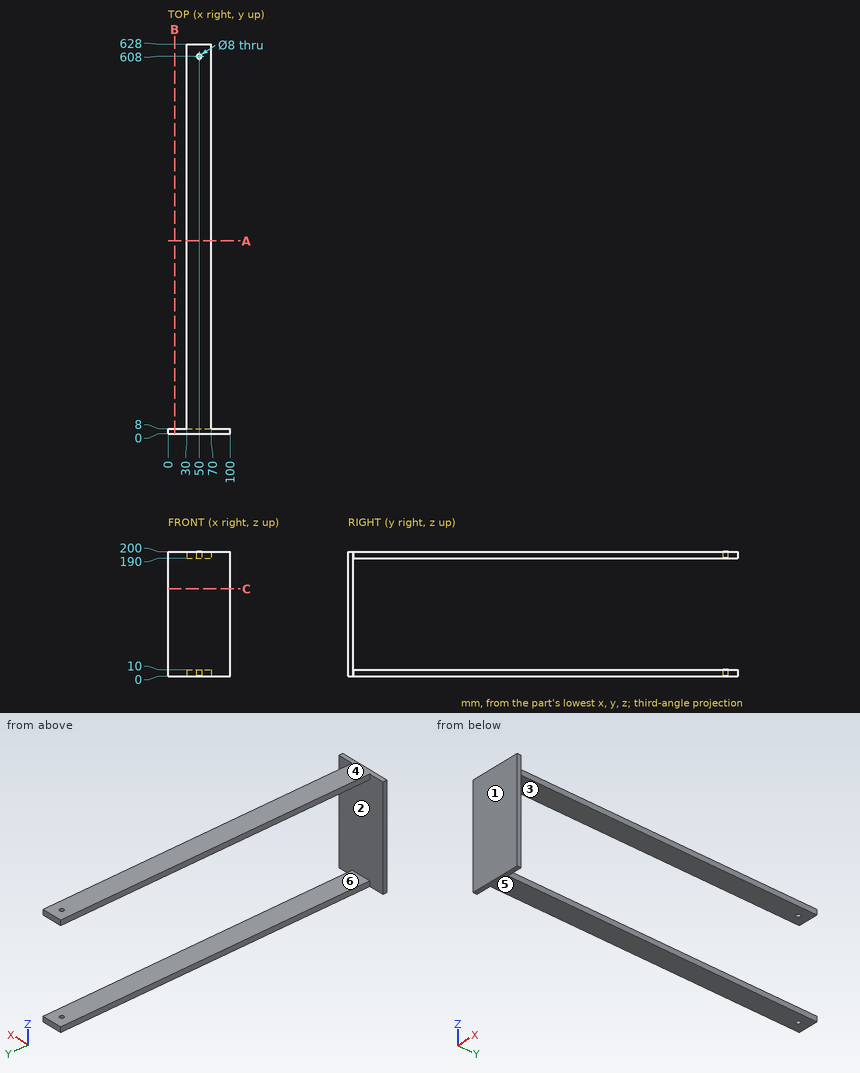
Check sheet for the drawn part. Datum: minimum x, y, z corner. Units: mm. A direction names the side the tool comes from. Round coordinates to 2 decimals unless told otherwise and drop trailing zeros. Order: outer loops, then holes, each group sorted by start corner. A loop starts at its lowest first (then second) coordinate and runs counter-clockwise, first axis right, second up. Notation, with made-up numbers: (25.25, 7.5) -> (83.25, 7.5) arc R28 ccw to (83.25, 25.5) -> close; hole circle Ø5 at (-40, 57). An arc over 180 degrees is marked (long way). Put each result on its own line as item: value. Start each with the question number.
(1) Material ranges on line 1 along Z through (x, y) = (59, 138); line 2 along Y through (x, z) = (50, 5); line 3 along Y through (x, z) = (25, 168.5), recorded low to high.
(2) Tool access check on the marked faces 5 and 6. Record the directions out of +Z, -Z, +X, -X, +Y, -Y that give a thin tool (end or side, any length) a straight path to the whole face; none if there is none.
(3) Draft check along Z on the marked faces 1, 2, 3 and 4. Enter one of: +Z half, -Z half, draft (parallel to the pull), parting line (faces both ways), or undercut.
(4) Section check A-A (y = 311). Enter the section's corners in (x, z).
(5) Depth check by flat-ended pin: pin 1 Ø1.5 at (x, z) = (54, 97.5) entering from +Y; pin 2 Ø5 at (y, z) = (400.5, 5) entering from -X; pin 3 Ø8 at (y, z) = (413, 195) entering from +X. Enter the tip coordinate at first touch or a pass-through.
(6) Section check B-B (x = 10.5). Enter the section's corners in (y, z).
(7) Section check C-C (z = 140.5). Enter the section's corners in (x, y).
Completed:
1. line 1: z = 0 to 10, 190 to 200
1. line 2: y = 0 to 604, 612 to 628
1. line 3: y = 0 to 8
2. face 5: -Z, +X, -X, +Y, -Y
2. face 6: +X, -X, +Y
3. face 1: draft
3. face 2: undercut
3. face 3: undercut
3. face 4: +Z half
4. outline: (30, 0) -> (70, 0) -> (70, 10) -> (30, 10) -> close; (30, 190) -> (70, 190) -> (70, 200) -> (30, 200) -> close
5. pin 1: stops at y = 8
5. pin 2: stops at x = 30
5. pin 3: stops at x = 70
6. outline: (0, 0) -> (8, 0) -> (8, 200) -> (0, 200) -> close
7. outline: (0, 0) -> (100, 0) -> (100, 8) -> (0, 8) -> close
